```python
from build123d import *

# Parameters (mm, degrees)
F2_DEPTH = 50.8
F1_R     = 12.7
F3_DEPTH = 50.8
F4_R     = 25.4
F4_R_2   = 12.7
F5_DEPTH = 50.8


# Not quite as in the source:
# - ends of sketch curves that miss each other by under 0.0002 mm in the source are joined


with BuildPart() as f2:
    # F0 (on Front) → F2 (new body)
    with BuildSketch(Plane.XZ):
        Polygon((0, 15.1726854965), (0, 0), (88.9, 0), (88.9, 15.1726854965), (38.1, 15.1726854965), align=None)
    extrude(amount=-F2_DEPTH)

    # F1 (on Top) → F3 (intersect)
    with BuildSketch(Plane.XY):
        with BuildLine():
            ThreePointArc((25.4023582082, 0), (43.3628704503, 7.4394877579), (50.8023582082, 25.4))
            ThreePointArc((50.8023582082, 25.4), (50.8017686493, 25.5730584989), (50.8, 25.7461089641))
            ThreePointArc((50.8, 25.7461089641), (43.2400827311, 43.4824661992), (25.4023582082, 50.8))
            ThreePointArc((25.4023582082, 50.8), (25.4011791041, 50.7999999726), (25.4, 50.7999998905))
            ThreePointArc((25.4, 50.7999998905), (0.0023582082, 25.4), (25.4, 1.095e-07))
            ThreePointArc((25.4, 1.095e-07), (25.4011791041, 2.74e-08), (25.4023582082, 0))
        make_face()
        with Locations((25.4023582082, 25.4)):
            Circle(F1_R, mode=Mode.SUBTRACT)
        with BuildLine():
            ThreePointArc((50.8, 25.7461089641), (50.8017686493, 25.5730584989), (50.8023582082, 25.4))
            ThreePointArc((50.8023582082, 25.4), (43.3628704503, 7.4394877579), (25.4023582082, 0))
            Line((25.4023582082, 0), (51.1508577362, 0))
            Line((51.1508577362, 0), (63.5, 0))
            Line((63.5, 0), (88.9, 25.4))
            Line((88.9, 25.4), (88.9, 50.8))
            Line((88.9, 50.8), (50.4585755345, 50.8))
            Line((50.4585755345, 50.8), (25.4023582082, 50.8))
            ThreePointArc((25.4023582082, 50.8), (43.2400827311, 43.4824661992), (50.8, 25.7461089641))
        make_face()
        with BuildLine():
            ThreePointArc((0, 25.4), (7.4394877579, 7.4394877579), (25.4, 0))
            ThreePointArc((25.4, 0), (0.0023582082, 25.4), (25.4, 50.7999998905))
            ThreePointArc((25.4, 50.7999998905), (7.4394877579, 43.3605122421), (0, 25.4))
        make_face()
    extrude(amount=F3_DEPTH, mode=Mode.INTERSECT)

    # F4 (on Top) → F5 (join)
    with BuildSketch(Plane.XY):
        with Locations((25.4, 25.1621566713)):
            Circle(F4_R)
        with Locations((25.4, 25.1621566713)):
            Circle(F4_R_2, mode=Mode.SUBTRACT)
    extrude(amount=F5_DEPTH)


solid = f2.part
```
Input: part model. Units: mm. Frame: model coordinates. A direction names the side the tool comes from. Give positions to 0.01 mm unless a question says otherwise; leave off trailing zeros. Order: outer loops, then holes, each group sorted by start corner. A loop starts at its lowest first (then second) coordinate and runs counter-clockwise, first axis right, second up.
1. Cut plane C-C (z = 6). Return loops of the section in (x, y).
Computed:
outline: (0, 25.28) arc R25.4 ccw to (28.87, 0) - (63.5, 0) - (88.9, 25.4) - (88.9, 50.8) - (25.4, 50.8) arc R25.4 ccw to start; hole (12.7, 25.41) arc R12.7 ccw to (38.1, 25.16) arc R12.7 ccw to start
2. Draft query along Y for faces 3 (the face through (23.747, 37.754, 30.689)), 4 (the face through (88.9, 38, 7)), 5 (the face through (19.894, 0.366, 30.689)), 6 (the face through (24.999, 12.706, 7.48)). Return one class per face: released by +Y, released by -Y, zero draft, split by the parting line, or undercut.
Computed:
face 3: undercut
face 4: zero draft
face 5: split by the parting line
face 6: undercut
3. Cut plane D-D (y = 4). Return loops of the section in (x, z), and give its area (3 significant figures).
Computed:
outline: (11.35, 0) - (67.5, 0) - (67.5, 15.17) - (39.45, 15.17) - (39.45, 50.8) - (11.35, 50.8) - close
area: 1,850 mm2
4. Cut plane A-A (y = 33). Return loops of the section in (x, z).
Computed:
outline: (1.16, 0) - (15.41, 0) - (15.41, 50.8) - (1.24, 50.8) - (1.24, 15.17) - (1.16, 15.17) - close; (35.39, 0) - (88.9, 0) - (88.9, 15.17) - (49.56, 15.17) - (49.56, 50.8) - (35.39, 50.8) - close
5. Line query: probe 1 along Y at (x, z) = (25.4, 19); probe 2 along Z at (x, y) = (67, 21); probe 3 along Y at (x, z) = (53.5, 13). Output: solid intervals per line, ascending.
Computed:
probe 1: y = -0.24 to 12.46, 37.86 to 50.56
probe 2: z = 0 to 15.17
probe 3: y = 0 to 50.8
6. Set-up query: faces 1 (the face through (46, 0, 8)), 2 (the face through (57, 50.8, 8)). Return all of +Z, -Z, +X, -X, +Y, -Y with unobstructed straight access to the full face (end or side cutting, diameter ignored); none if empty.
Computed:
face 1: +Z, -Z, +X, -Y
face 2: +Z, -Z, +X, -X, +Y
7. Cut plane B-B (x = 17). Return loops of the section in (y, z).
Computed:
outline: (1.19, 0) - (15.88, 0) - (15.88, 15.17) - (15.64, 15.17) - (15.64, 50.8) - (1.19, 50.8) - close; (34.69, 0) - (49.37, 0) - (49.37, 15.17) - (49.13, 15.17) - (49.13, 50.8) - (34.69, 50.8) - close
8. Pin query (flat end, axial travel): pin 1 Ø1.5 at (y, z) = (36.5, 14.5) entering from -X; pin 2 Ø8 at (y, z) = (12.5, 42.5) entering from -X; pin 3 Ø2 at (y, z) = (24, 16.5) entering from -X. Return the tip coordinate at first contact, or that it passes through.
Computed:
pin 1: stops at x = 2.2
pin 2: stops at x = 1.52
pin 3: stops at x = 0
